Build history of the part. All positions in model axes, mm. Give positions to 0.01 mm unless a question says otherwise; leave off trailing zeros. Write each loop counter-clockwise with the first axis right and the second up, starting at its lowest first coordinate (ties: lowest second). Pieces come first, ordered by that corner, then holes. Notation, with made-up numbers: M -34.5,19.25 L -26.5,19.25 A20 cw -26.5,23.25 Z; hole C -6,87.5 d3. An arc over 180 degrees is marked long. Return JSON: item names as keys, results as strings. Group by question number.
Q1. Flat gauge pins, fed straight in: pin 1 Ø2 at (x, y) = (48.5, -1.5) entering from +Z; pin 2 Ø1.3 at (x, z) = (33, 4) entering from -Y; pin 3 Ø1.3 at (x, z) = (30, 4) entering from +Y. Where does each tip first touch, or does it go through?
Q2. Wall check: probe 1 along X at (y, z) = (-4, 2.75); probe 2 along Y at (x, z) = (43, -0.25); probe 3 along X at (y, z) = (-1, 4). Give the ranges that are in metal, low to high.
Q3. Band-saw the part on B-B, the plane x = 51.5. Give the cut face in (y, z).
Q4. Band-saw the part on A-A, the plane y = 0. Give the cut face in (x, z), then the cut area to 3 significant figures.
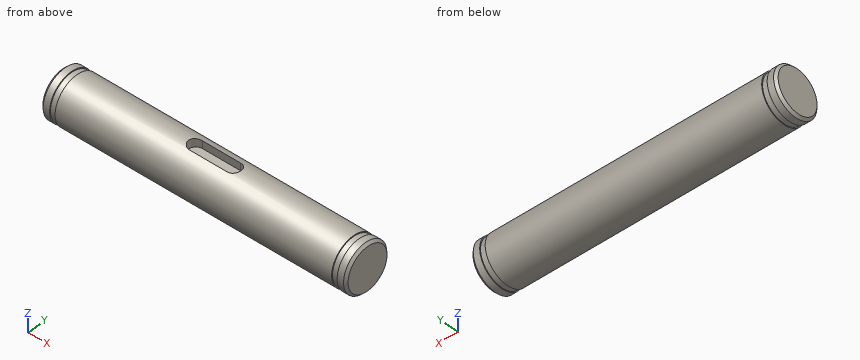
Autodesk Inventor part; units mm, degrees
ref_plane "COMBINATION_MODULE_XY" through (0, 0, 0) normal (1, 0, 0) x (0, 0, -1)
ref_plane "COMBINATION_MODULE_YZ" through (0, 0, 0) normal (0, 0, -1) x (0, 1, 0)
ref_plane "COMBINATION_MODULE_ZX" through (0, 0, 0) normal (0, 1, 0) x (1, 0, 0)
sketch "Sketch_1" plane through (0, 0, 0) normal (0, 0, 1) x (1, 0, 0)
  line L0 (64, 0) -> (0, 0)
  line L1 (0, 0) -> (0, 4.5)
  line L2 (0, 4.5) -> (0.5, 5)
  line L3 (0.5, 5) -> (63.5, 5)
  line L4 (63.5, 5) -> (64, 4.5)
  line L5 (64, 4.5) -> (64, 0)
  line L6 (64, 0) -> (0, 0)
revolve "Revolution1" add sketch "Sketch_1" angle 360 about axis through (64, 0, 0) along (1, 0, 0)
sketch "_____10" plane through (0, 0, 5) normal (0, 0, 1) x (1, 0, 0)
  arc A0 (28, 1.5) -> (28, -1.5) centre (28, 0) ccw
  line L0 (28, -1.5) -> (36, -1.5)
  arc A1 (36, -1.5) -> (36, 1.5) centre (36, 0) ccw
  line L1 (36, 1.5) -> (28, 1.5)
extrude "Extrusion1" cut sketch "_____10" against normal blind 1.8
sketch "_____5" plane through (3, 0, 0) normal (1, 0, 0) x (0, 0, -1)
  circle A0 centre (0, 0) radius 10
  circle A1 centre (0, 0) radius 4.8
extrude "Extrusion2" cut sketch "_____5" against normal blind 1.15
sketch "_____6" plane through (61, 0, 0) normal (1, 0, 0) x (0, 0, -1)
  circle A0 centre (0, 0) radius 10
  circle A1 centre (0, 0) radius 4.8
extrude "Extrusion3" cut sketch "_____6" along normal blind 1.15
ref_plane "COMBINATION_MODULE_XY" through (0, 0, 0) normal (1, 0, 0) x (0, 0, -1)
ref_plane "COMBINATION_MODULE_YZ" through (0, 0, 0) normal (0, 0, -1) x (0, 1, 0)
ref_plane "COMBINATION_MODULE_ZX" through (0, 0, 0) normal (0, 1, 0) x (1, 0, 0)
ref_plane "to_ring_b_XY" through (2.425, 0, 0) normal (1, 0, 0) x (0, 0, -1)
ref_plane "to_ring_b_YZ" through (2.425, 0, 0) normal (0, 0, -1) x (0, 1, 0)
ref_plane "to_ring_b_ZX" through (2.425, 0, 0) normal (0, 1, 0) x (1, 0, 0)
ref_plane "to_ring_s_XY" through (61.575, 0, 0) normal (1, 0, 0) x (0, 0, -1)
ref_plane "to_ring_s_YZ" through (61.575, 0, 0) normal (0, 0, -1) x (0, 1, 0)
ref_plane "to_ring_s_ZX" through (61.575, 0, 0) normal (0, 1, 0) x (1, 0, 0)
properties part number "NSFMRRA10-64-B3-S3-KC26.5-A11(000_000)_s"
From the geometry:
{
 "1": {"pin 1": "stops at z = 4.97", "pin 2": "stops at y = -3.71", "pin 3": "stops at y = 3.71"},
 "2": {"probe 1": "x = 0.35 to 1.85, 3 to 61, 62.15 to 63.65", "probe 2": "y = -4.99 to 4.99", "probe 3": "x = 0 to 26.88, 37.12 to 64"},
 "3": {"outline": "C 0,0 d10"},
 "4": {"outline": "M 0,-4.5 L 0.5,-5 L 1.85,-5 L 1.85,-4.8 L 3,-4.8 L 3,-5 L 61,-5 L 61,-4.8 L 62.15,-4.8 L 62.15,-5 L 63.5,-5 L 64,-4.5 L 64,4.5 L 63.5,5 L 62.15,5 L 62.15,4.8 L 61,4.8 L 61,5 L 37.5,5 L 37.5,3.2 L 26.5,3.2 L 26.5,5 L 3,5 L 3,4.8 L 1.85,4.8 L 1.85,5 L 0.5,5 L 0,4.5 Z", "area": "619 mm^2"}
}
